Part print with two shaded views. Sizes in mm from the minimum x, y, z corner. A direction names the side the tool comes from. Round coordinates to 2 decimals unless told otherwise and drop trailing zeros. Loops run counter-clockwise (first coordinate to the right, second up) from the corner with the lowest first, then second, coordinate; pieces in that order, holes last. Notation, with made-up numbers: (-10, 27.5) - (20, 27.5) arc R16 ccw to (20, 48.5) - close; hole circle Ø1 at (59, 21.5). An arc over 180 degrees is marked (long way). Use a Markdown table: item, result.
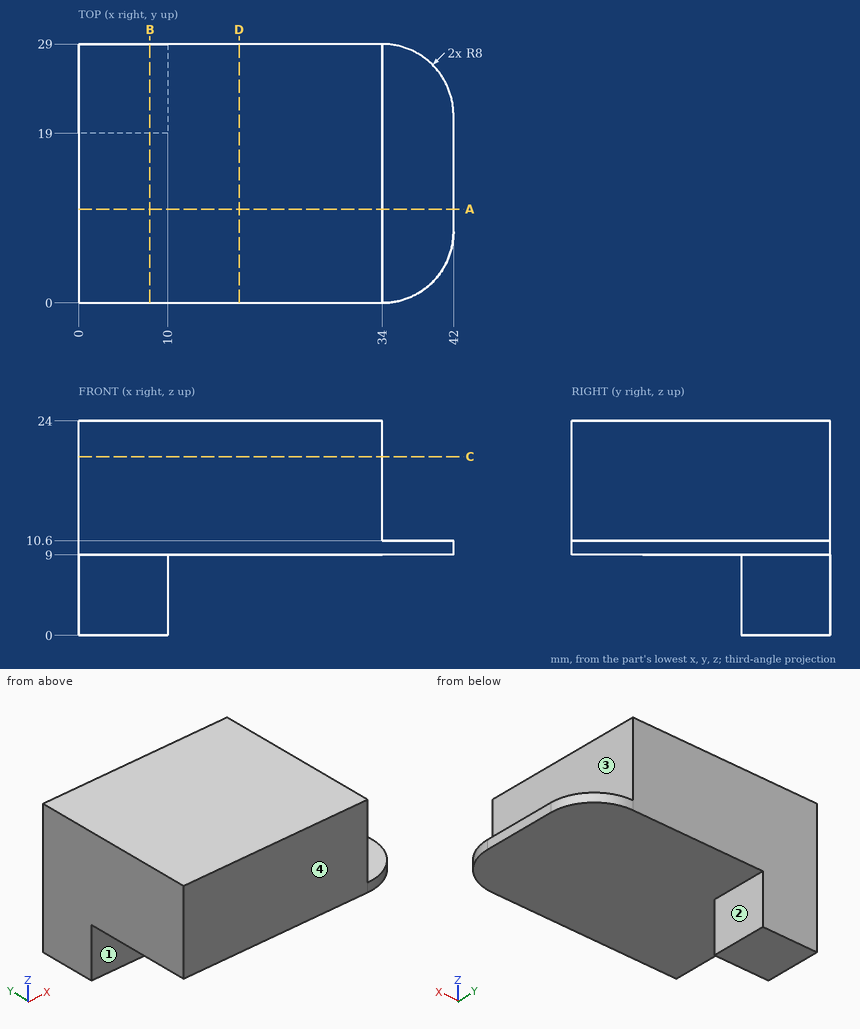
Q1. Which spindle directions (+Z, -Z, +X, -X, +Y, -Y) get a long thin tool onto all of the face, cutting with end or side? Do the marked faces 1, 2, 3 and 4. Say none if no direction does.
Results found:
| item | result |
|---|---|
| face 1 | -Z, +X, -X, -Y |
| face 2 | -Z, +X, +Y, -Y |
| face 3 | +Z, +X, +Y, -Y |
| face 4 | +Z, -Z, +X, -X, -Y |
Q2. Cut at D-D, the plane x = 18. List the corners of the cut face in (y, z).
Results found:
| item | result |
|---|---|
| outline | (0, 9) - (29, 9) - (29, 24) - (0, 24) - close |
Q3. Cut at A-A, the plane y = 10.5. List the corners of the cut face in (x, z), plus the area to 3 significant figures.
Results found:
| item | result |
|---|---|
| outline | (0, 9) - (42, 9) - (42, 10.6) - (34, 10.6) - (34, 24) - (0, 24) - close |
| area | 523 mm2 |
Q4. Cut at B-B, the plane x = 8. List the corners of the cut face in (y, z).
Results found:
| item | result |
|---|---|
| outline | (0, 9) - (19, 9) - (19, 0) - (29, 0) - (29, 24) - (0, 24) - close |
Q5. Probe line 1 (Z direction, x = 37.5, y = 16.5); line 2 (Z direction, x = 26, y = 19); line 3 (X direction, y = 5.25, z = 18.75). List the from-to ranges inside material, lowest first.
Results found:
| item | result |
|---|---|
| line 1 | z = 9 to 10.6 |
| line 2 | z = 9 to 24 |
| line 3 | x = 0 to 34 |
Q6. Drop flat-ended pins along their axis: pin 1 (1 mm diameter, centred on x = 29.5, y = 10.5, fed in from -Z); pin 2 (10 mm diameter, centred on y = 26, z = 5.5, fed in from +X); pin 3 (10 mm diameter, centred on x = 24.5, z = 17.5, fed in from -Y); pin 4 (4.5 mm diameter, centred on x = 5, z = 6.5, fed in from -Y). Give the stop position or say it passes through.
Results found:
| item | result |
|---|---|
| pin 1 | stops at z = 9 |
| pin 2 | stops at x = 41.87 |
| pin 3 | stops at y = 0 |
| pin 4 | stops at y = 19 |
Q7. Cut at C-C, the plane z = 20. List the corners of the cut face in (x, y).
Results found:
| item | result |
|---|---|
| outline | (0, 0) - (34, 0) - (34, 29) - (0, 29) - close |
